```python
from build123d import *

# Parameters (mm, degrees)
F0_W     = 207
F0_H     = 116
F1_DEPTH = 6
F2_W     = 167
F2_H     = 102
F3_DEPTH = 25
F4_R     = 1.75
F5_DEPTH = 25
F6_R     = 5
F7_R     = 1
F8_W     = 10
F8_H     = 60
F9_DEPTH = 3


with BuildPart() as f1:
    # F0 (on Top) → F1 (new body)
    with BuildSketch(Plane.XY):
        with Locations((103.5, -58)):
            Rectangle(F0_W, F0_H)
    extrude(amount=F1_DEPTH)

    # F2 (on face) → F3 (cut)
    with BuildSketch(Plane.XY):
        with Locations((113, -58)):
            Rectangle(F2_W, F2_H)
    extrude(amount=F3_DEPTH, mode=Mode.SUBTRACT)

    # F4 (on face) → F5 (cut)
    with BuildSketch(Plane(origin=(0, 0, 0), x_dir=(1, 0, 0), z_dir=(0, 0, -1))):
        with Locations((200, 7)):
            Circle(F4_R)
        with Locations((200, 109)):
            Circle(F4_R)
        with Locations((25, 109)):
            Circle(F4_R)
        with Locations((25, 7)):
            Circle(F4_R)
    extrude(amount=-F5_DEPTH, mode=Mode.SUBTRACT)

    # F6
    f6_edges = [f1.edges().sort_by_distance(p)[0] for p in [
        (207, 0, 3),
        (207, -116, 3),
        (0, -116, 3),
        (0, 0, 3),
    ]]
    fillet(f6_edges, radius=F6_R)

    # F7
    f7_edges = [f1.edges().sort_by_distance(p)[0] for p in [
        (207, -58, 0),
        (198.25, -7, 0),
    ]]
    fillet(f7_edges, radius=F7_R)

    # F8 (on face) → F9 (cut)
    with BuildSketch(Plane.XY.offset(6)):
        with Locations((24.5, -58)):
            Rectangle(F8_W, F8_H)
    extrude(amount=-F9_DEPTH, mode=Mode.SUBTRACT)


solid = f1.part
```
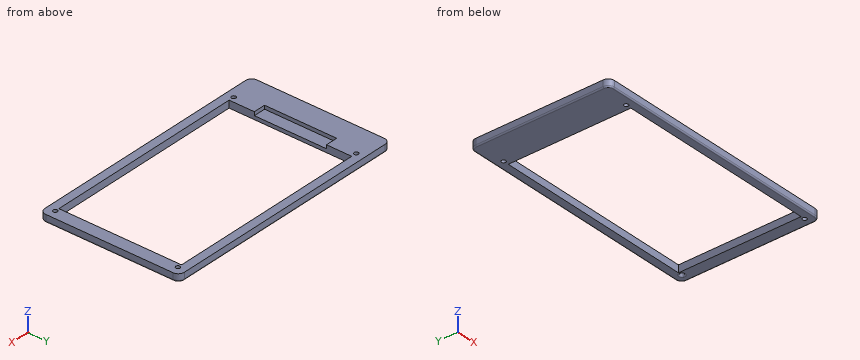
Work out the finished part from the listing and answer in its coordinate system (mm). Coordinates: 2 decimals unless noted, no trailing zeros. Loops run counter-clockwise (first coordinate to the right, second up) from the corner with the lowest first, then second, coordinate; pieces in that order, holes last. Notation, with made-up numbers: M 59.25,44.5 L 63.25,44.5 A26 cw 63.25,61.5 Z; hole C 31,34.25 d1. An arc over 180 degrees is marked long. Use CSV: the item, a comma, the result in double quotes. Start each with the question number.
(1) Given pin 1 Ø4 at (x, y) = (200, -7) entering from +Z; pin 2 Ø3 at (x, y) = (26.5, -43) entering from +Z, each flat-ended and moving along its own axis, determine where each tip first touches the part or whether it passes through.
(2) Find section A-A, the plane x = 193. Give the vertices of the cut face in (y, z).
(3) Find section B-B, the plane y = -98. Give the vertices of the cut face in (x, z), then the cut area to 3 significant figures.
(4) Find section D-D, the plane y = -62.5. Give the vertices of the cut face in (x, z), then the cut area to 3 significant figures.
(5) Find section C-C, the plane z = 3.95. Give the vertices of the cut face in (x, y).
(6) Consider line 1 (Y direction, x = 25, z = 2.4); line 2 (Y direction, x = 25, z = 4.65); line 3 (X direction, y = -28, z = 2.2). Determine where each line is inside the solid, lowest interval first.
Recorded:
1,pin 1,"stops at z = 6"
1,pin 2,"stops at z = 3"
2,outline,"M -116,1 A1 ccw -115,0 L -109,0 L -109,6 L -116,6 Z; M -7,0 L -1,0 A1 ccw 0,1 L 0,6 L -7,6 Z"
3,outline,"M 0,1 A1 ccw 1,0 L 29.5,0 L 29.5,6 L 0,6 Z; M 196.5,0 L 206,0 A1 ccw 207,1 L 207,6 L 196.5,6 Z"
3,area,"240 mm^2"
4,outline,"M 0,1 A1 ccw 1,0 L 29.5,0 L 29.5,3 L 19.5,3 L 19.5,6 L 0,6 Z; M 196.5,0 L 206,0 A1 ccw 207,1 L 207,6 L 196.5,6 Z"
4,area,"210 mm^2"
5,outline,"M 0,-111 A5 ccw 5,-116 L 202,-116 A5 ccw 207,-111 L 207,-5 A5 ccw 202,0 L 5,0 A5 ccw 0,-5 Z; hole M 19.5,-88 L 29.5,-88 L 29.5,-109 L 196.5,-109 L 196.5,-7 L 29.5,-7 L 29.5,-28 L 19.5,-28 Z; hole C 25,-109 d3.5; hole C 25,-7 d3.5; hole C 200,-109 d3.5; hole C 200,-7 d3.5"
6,line 1,"y = -116 to -110.75, -107.25 to -8.75, -5.25 to 0"
6,line 2,"y = -116 to -110.75, -107.25 to -88, -28 to -8.75, -5.25 to 0"
6,line 3,"x = 0 to 29.5, 196.5 to 207"
